```python
from build123d import *

# Parameters (mm, degrees)
ESQUISSE1_R        = 1.5
BOSS_EXTRU_1_DEPTH = 5
CONG_1_R           = 5
CONG_3_START       = -1
CONG_3_DEPTH       = 7
CONG_3_2_DEPTH     = 5


with BuildPart() as part:
    # Esquisse1 → Boss.-Extru.1 (new body)
    with BuildSketch(Plane.XY):
        Polygon((20, 0), (20, 7), (15, 7), (15, 12), (20, 12), (20, 20), (12, 20), (12, 39), (20, 39), (20, 47), (15, 47), (15, 52), (20, 52), (20, 58), (-20, 58), (-20, 52), (-15, 52), (-15, 47), (-20, 47), (-20, 39), (-12, 39), (-12, 20), (-20, 20), (-20, 12), (-15, 12), (-15, 7), (-20, 7), (-20, 0), (-15, 0), (-15, -5), (-20, -5), (-20, -11), (20, -11), (20, -5), (15, -5), (15, 0), align=None)
        with Locations((0, 49.5)):
            Circle(ESQUISSE1_R, mode=Mode.SUBTRACT)
        with Locations((0, 9.5)):
            Circle(ESQUISSE1_R, mode=Mode.SUBTRACT)
    extrude(amount=BOSS_EXTRU_1_DEPTH)

    # Congé1
    cong_1_edges = [part.edges().sort_by_distance(p)[0] for p in [
        (-20, 58, 2.5),
        (20, 58, 2.5),
        (20, -11, 2.5),
        (-20, -11, 2.5),
    ]]
    fillet(cong_1_edges, radius=CONG_1_R)

    # Congé3: read off the stored shape, not the designer's step
    # Congé3 outline → Congé3 (cut)
    with BuildSketch(Plane.XY.offset(CONG_3_START)):
        with BuildLine():
            Line((20, 20), (16, 20))
            ThreePointArc((16, 20), (18.828427125, 18.828427125), (20, 16))
            Line((20, 16), (20, 20))
        make_face()
        with BuildLine():
            ThreePointArc((20, 43), (18.828427125, 40.171572875), (16, 39))
            Line((16, 39), (20, 39))
            Line((20, 39), (20, 43))
        make_face()
        with BuildLine():
            Line((-20, 39), (-16, 39))
            ThreePointArc((-16, 39), (-18.828427125, 40.171572875), (-20, 43))
            Line((-20, 43), (-20, 39))
        make_face()
        with BuildLine():
            ThreePointArc((-20, 16), (-18.828427125, 18.828427125), (-16, 20))
            Line((-16, 20), (-20, 20))
            Line((-20, 20), (-20, 16))
        make_face()
    extrude(amount=CONG_3_DEPTH, mode=Mode.SUBTRACT)

    # Cong_3 2 outline → Cong_3 2 (add)
    with BuildSketch(Plane.XY):
        with BuildLine():
            Line((12, 39), (12, 35))
            ThreePointArc((12, 35), (13.171572875, 37.828427125), (16, 39))
            Line((16, 39), (12, 39))
        make_face()
        with BuildLine():
            ThreePointArc((16, 20), (13.171572875, 21.171572875), (12, 24))
            Line((12, 24), (12, 20))
            Line((12, 20), (16, 20))
        make_face()
        with BuildLine():
            ThreePointArc((-16, 39), (-13.171572875, 37.828427125), (-12, 35))
            Line((-12, 35), (-12, 39))
            Line((-12, 39), (-16, 39))
        make_face()
        with BuildLine():
            ThreePointArc((-12, 24), (-13.171572875, 21.171572875), (-16, 20))
            Line((-16, 20), (-12, 20))
            Line((-12, 20), (-12, 24))
        make_face()
    extrude(amount=CONG_3_2_DEPTH)


solid = part.part
```
For this review, take the finished solid that the model builds, in its own axes (mm). A direction names the side the tool comes from. Coordinates: 2 decimals unless noted, no trailing zeros. Loops run counter-clockwise (first coordinate to the right, second up) from the corner with the lowest first, then second, coordinate; pieces in that order, holes last. Notation, with made-up numbers: (-14, 81) - (43, 81) arc R22 cw to (43, 97) - close; hole circle Ø6 at (37, -12). An arc over 180 degrees is marked (long way). Use one line per item in the form item = value. Start each with the question number.
1) For faces 1 (the face through (-18, 12, 2)), 2 (the face through (-20, 4, 2)), 3 (the face through (17, 0, 2)), list the 3-axis set-ups (+Z, -Z, +X, -X, +Y, -Y) from which the entire face can be reached by the end or side of a thin tool; tool diameter is ignored.
2) Take a section at C-C (z = 1.15). State how many separate pieces and enclosed holes the cut face has, plus the area to 3 significant figures.
3) For pin 1 (2.5 mm diameter, centred on y = 10.5, z = 2.5, fed in from +X); pin 2 (1.5 mm diameter, centred on x = -17, z = 1.5, fed in from +Y); pin 3 (2.5 mm diameter, centred on y = 10, z = 3, fed in from -X); pin 4 (2.5 mm diameter, centred on x = 0, y = 49.5, fed in from -Z), all flat-tipped, find the tip position at first contact; note any pin that passes through.
4) Take a section at A-A (y = 9.5). State the section outline as (x, z) points.
5) To check wall thickness, follow probe 1 along Y at (x, z) = (0, 1.4); probe 2 along Y at (x, z) = (-0.5, 4.35); probe 3 along Y at (x, z) = (-17, 3.45). State the ranges of each line that lie inside material, in increasing order. Write a range as from..to.
6) Take a section at D-D (y = 33.5). State the section outline as (x, z) points.
7) Take a section at B-B (x = 0). State the section outline as (y, z) points, plus the area to 3 significant figures.
8) Draft analysis for pull direction Y (two halves, no side actions). For faces 4 (the face through (-18, 57, 3)), 5 (the face through (-18, -10, 3)), 6 (the face through (0, 48, 2)), state which applies: released by +Y, released by -Y, zero draft, split by the parting line, or undercut.
From the geometry:
q1.face_1 = +Z, -Z, -X
q1.face_2 = +Z, -Z, -X, +Y, -Y
q1.face_3 = +Z, -Z, +X
q2.separate_pieces = 1
q2.enclosed_holes = 2
q2.area = 2,270 mm2
q3.pin_1 = 15
q3.pin_2 = 57.84
q3.pin_3 = -15
q3.pin_4 = through
q4.outline = (-15, 0) - (-1.5, 0) - (-1.5, 5) - (-15, 5) - close; (1.5, 0) - (15, 0) - (15, 5) - (1.5, 5) - close
q5.probe_1 = -11..8, 11..48, 51..58
q5.probe_2 = -11..8.09, 10.91..48.09, 50.91..58
q5.probe_3 = -10.58..-5, 0..7, 12..19.87, 39.13..47, 52..57.58
q6.outline = (-12, 0) - (12, 0) - (12, 5) - (-12, 5) - close
q7.outline = (-11, 0) - (8, 0) - (8, 5) - (-11, 5) - close; (11, 0) - (48, 0) - (48, 5) - (11, 5) - close; (51, 0) - (58, 0) - (58, 5) - (51, 5) - close
q7.area = 315 mm2
q8.face_4 = released by +Y
q8.face_5 = released by -Y
q8.face_6 = undercut
